Autodesk Inventor part; units mm, degrees
ref_plane "YZ Plane" through (0, 0, 0) normal (1, 0, 0) x (0, 1, 0)
ref_plane "XZ Plane" through (0, 0, 0) normal (0, 1, 0) x (-1, 0, 0)
ref_plane "XY Plane" through (0, 0, 0) normal (0, 0, 1) x (1, 0, 0)
sketch "スケッチ1" plane through (0, 0, 0) normal (0, 0, 1) x (1, 0, 0)
  line L0 (0, 0) -> (239.9998, 0)
  line L1 (239.9998, 0) -> (239.9998, 239.9998)
  line L2 (239.9998, 239.9998) -> (0, 239.9998)
  line L3 (0, 239.9998) -> (0, 0)
  line L4 (0, 239.9998) -> (239.9998, 0)
  line L5 (-178.706, 178.706) -> (151.9787, -151.9787)
  dimension "d16" = 45
  dimension "d17" = 169.7055
extrude "プレート1" add sketch "スケッチ1" along normal blind 1.5 contours L3 L4 L0
sketch "スケッチ2" plane through (0, 0, 1.5) normal (0, 0, 1) x (1, 0, 0)
  line L0 (90, 33.5) -> (110, 33.5)
  line L1 (110, 33.5) -> (110, 86.5)
  line L2 (110, 86.5) -> (90, 86.5)
  line L3 (90, 86.5) -> (90, 33.5)
  line L4 (90, 33.5) -> (110, 86.5) construction
  line L5 (110, 33.5) -> (90, 86.5) construction
  line L6 (239.9998, 0) -> (0, 0)
  line L7 (0, 0) -> (0, 239.9998)
  line L8 (134, 30) -> (66, 30)
  line L9 (66, 30) -> (66, 90)
  line L10 (66, 90) -> (134, 90)
  line L11 (134, 90) -> (134, 30)
  line L12 (134, 30) -> (66, 90) construction
  line L13 (66, 30) -> (134, 90) construction
  point P0 (100, 60)
  dimension "d3" = 20
  dimension "d4" = 53
  dimension "d5" = 60
  dimension "d6" = 100
  dimension "d14" = 60
  dimension "d15" = 68
hole "穴1" at (90, 33.5, 1.5) at (110, 33.5, 1.5) at (90, 86.5, 1.5) at (110, 86.5, 1.5) at (66, 30, 1.5) at (134, 30, 1.5) at (66, 90, 1.5) direction (0, 0, -1) diameter 5.2 depth 1.5 tip angle 118
fillet "フィレット1" radius 2 3 edges at (0, 239.9998, 0.75) (0, 0, 0.75) (239.9998, 0, 0.75)
sketch "スケッチ3" plane through (0, 0, 1.5) normal (0, 0, 1) x (1, 0, 0)
  circle A0 centre (66, 90) radius 2.6
  line L0 (0, 2) -> (0, 235.1714)
  point P0 (0, 0)
  point P1 (90, 117)
  point P2 (80, 117)
  dimension "d19" = 10
  dimension "d20" = 27
  dimension "d21" = 80
hole "穴2" at (90, 117, 1.5) at (80, 117, 1.5) direction (0, 0, -1) diameter 3.242 depth 11.8 tip angle 118
sketch "スケッチ4" plane through (0, 0, 1.5) normal (0, 0, 1) x (1, 0, 0)
  circle A0 centre (90, 117) radius 1.621
  circle A1 centre (80, 117) radius 1.621
  arc A2 (235.1714, 0) -> (236.5856, 3.4142) centre (235.1714, 2) ccw
  line L0 (3.4142, 236.5856) -> (236.5856, 3.4142)
  arc A3 (3.4142, 236.5856) -> (0, 235.1714) centre (2, 235.1714) ccw
  line L1 (0, 2) -> (0, 235.1714)
  arc A4 (0, 2) -> (2, 0) centre (2, 2) ccw
  line L2 (235.1714, 0) -> (2, 0)
  circle A5 centre (134, 30) radius 2.6
  circle A6 centre (110, 86.5) radius 2.6
  circle A7 centre (110, 33.5) radius 2.6
  circle A8 centre (90, 33.5) radius 2.6
  circle A9 centre (90, 86.5) radius 2.6
  circle A10 centre (66, 30) radius 2.6
  circle A11 centre (66, 90) radius 2.6
  line L3 (10, 10) -> (10, 215.8577)
  line L4 (10, 215.8577) -> (215.8577, 10)
  line L5 (215.8577, 10) -> (10, 10)
  point P0 (0, 0)
  point P1 (205, 10)
  point P2 (35, 10)
  point P3 (10, 35)
  point P4 (10, 205)
  point P5 (120, 10)
  point P6 (10, 120)
  dimension "d29" = 10
  dimension "d30" = 25
  dimension "d31" = 25
  dimension "d32" = 170
  dimension "d33" = 170
  dimension "d34" = 85
  dimension "d35" = 85
hole "穴3" at (205, 10, 1.5) at (35, 10, 1.5) at (10, 35, 1.5) at (10, 205, 1.5) at (120, 10, 1.5) at (10, 120, 1.5) direction (0, 0, -1) diameter 4.2 depth 1.5 tip angle 118
sketch "スケッチ6" plane through (0, 0, 1.5) normal (0, 0, 1) x (1, 0, 0)
  circle A0 centre (120, 10) radius 2.1
  circle A1 centre (10, 35) radius 2.1
  circle A2 centre (205, 10) radius 2.1
  circle A3 centre (35, 10) radius 2.1
  circle A4 centre (10, 205) radius 2.1
  circle A5 centre (10, 120) radius 2.1
  circle A6 centre (90, 117) radius 1.621
  circle A7 centre (80, 117) radius 1.621
  arc A8 (235.1714, 0) -> (236.5856, 3.4142) centre (235.1714, 2) ccw
  line L0 (3.4142, 236.5856) -> (236.5856, 3.4142)
  arc A9 (3.4142, 236.5856) -> (0, 235.1714) centre (2, 235.1714) ccw
  line L1 (0, 2) -> (0, 235.1714)
  arc A10 (0, 2) -> (2, 0) centre (2, 2) ccw
  line L2 (235.1714, 0) -> (2, 0)
  circle A11 centre (134, 30) radius 2.6
  circle A12 centre (110, 86.5) radius 2.6
  circle A13 centre (110, 33.5) radius 2.6
  circle A14 centre (90, 33.5) radius 2.6
  circle A15 centre (90, 86.5) radius 2.6
  circle A16 centre (66, 30) radius 2.6
  circle A17 centre (66, 90) radius 2.6
  line L3 (20, 20) -> (20, 191.7155)
  line L4 (20, 191.7155) -> (191.7155, 20)
  line L5 (191.7155, 20) -> (20, 20)
  point P0 (0, 0)
  point P1 (30, 30)
  dimension "d46" = 20
  dimension "d47" = 10
  dimension "d48" = 10
hole "穴4" at (30, 30, 1.5) direction (0, 0, -1) diameter 5.2 depth 1.5 tip angle 118
sketch "スケッチ7" plane through (0, 0, 1.5) normal (0, 0, 1) x (1, 0, 0)
  circle A0 centre (30, 30) radius 2.6
  circle A1 centre (120, 10) radius 2.1
  circle A2 centre (10, 35) radius 2.1
  circle A3 centre (205, 10) radius 2.1
  circle A4 centre (35, 10) radius 2.1
  circle A5 centre (10, 205) radius 2.1
  circle A6 centre (10, 120) radius 2.1
  circle A7 centre (90, 117) radius 1.621
  circle A8 centre (80, 117) radius 1.621
  arc A9 (235.1714, 0) -> (236.5856, 3.4142) centre (235.1714, 2) ccw
  line L0 (3.4142, 236.5856) -> (236.5856, 3.4142)
  arc A10 (3.4142, 236.5856) -> (0, 235.1714) centre (2, 235.1714) ccw
  line L1 (0, 2) -> (0, 235.1714)
  arc A11 (0, 2) -> (2, 0) centre (2, 2) ccw
  line L2 (235.1714, 0) -> (2, 0)
  circle A12 centre (134, 30) radius 2.6
  circle A13 centre (110, 86.5) radius 2.6
  circle A14 centre (110, 33.5) radius 2.6
  circle A15 centre (90, 33.5) radius 2.6
  circle A16 centre (90, 86.5) radius 2.6
  circle A17 centre (66, 30) radius 2.6
  circle A18 centre (66, 90) radius 2.6
  point P0 (0, 0)
extrude "押し出し2" add sketch "スケッチ7" against normal up to surface (1.5 mm away) contours A7 | A8 | A12 | A13 | A14 | A15 | A16 | A17 | A18
equation "\"d12\" = Thickness"
equation "\"d41\" = Thickness"
equation "\"d54\" = Thickness"
equation "\"d2\" = Thickness"
equation "\"BendRadius\" = Thickness"
equation "\"BendReliefWidth\" = Thickness"
equation "\"BendReliefDepth\" = 0.5 * Thickness"
equation "\"CornerReliefSize\" = 4 * Thickness"
equation "\"MinimumRemnant\" = 2 * Thickness"
equation "\"TransitionRadius\" = BendRadius"
equation "\"JacobiRadiusSize\" = BendRadius"
equation "\"GapSize\" = Thickness"
properties part number "Display_CCM_Mount_Top"
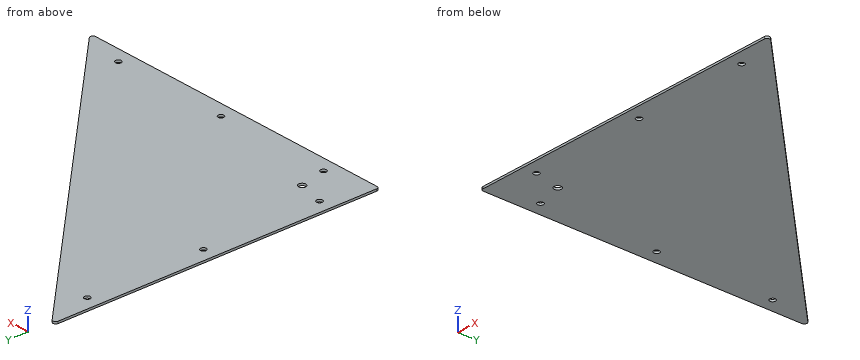
Source: CAD feature listing. Evaluate the final solid. Frame: model axes, mm. Round coordinates to 2 decimals unless told otherwise and drop trailing zeros. Loops run counter-clockwise (first coordinate to the right, second up) from the corner with the lowest first, then second, coordinate; pieces in that order, holes last. Notation, with made-up numbers: (73, 3) - (103, 3) arc R24 ccw to (103, 19) - close; hole circle Ø11 at (21.25, 35). An arc over 180 degrees is marked (long way). Write item = value, one per line. Start each with the question number.
(1) Section query C-C, the plane x = 80. Output: boundary loops of the cut face in (y, z), plus the area to 3 significant figures.
(2) Section query B-B, the plane y = 135.5. Output: boundary loops of the cut face in (x, z), plus the area to 3 significant figures.
(3) Pin query (flat end, axial travel): pin 1 (4 mm diameter, centred on x = 30, y = 30, fed in from +Z). Return the tip coordinate at first contact, or that it passes through.
(4) Ray query, line 1 along Y through (x, z) = (10, 0.3); line 2 along X through (y, z) = (10.5, 0.6); line 3 along X through (y, z) = (32, 1.45). Return the intervals inside material, ascending. Write a range as from..to.
(5) Section query A-A, the plane z = 1.25. Output: boundary loops of the cut face in (x, y), plus the area to 3 significant figures.
Conclusion:
q1.outline = (0, 0) - (160, 0) - (160, 1.5) - (0, 1.5) - close
q1.area = 240 mm2
q2.outline = (0, 0) - (104.5, 0) - (104.5, 1.5) - (0, 1.5) - close
q2.area = 157 mm2
q3.pin_1 = through
q4.line_1 = 0..32.9, 37.1..117.9, 122.1..202.9, 207.1..230
q4.line_2 = 0..32.96, 37.04..117.96, 122.04..202.96, 207.04..229.5
q4.line_3 = 0..28.34, 31.66..208
q5.outline = (0, 2) arc R2 ccw to (2, 0) - (235.17, 0) arc R2 ccw to (236.59, 3.41) - (3.41, 236.59) arc R2 ccw to (0, 235.17) - close; hole circle Ø4.2 at (10, 35); hole circle Ø4.2 at (10, 120); hole circle Ø4.2 at (10, 205); hole circle Ø5.2 at (30, 30); hole circle Ø4.2 at (35, 10); hole circle Ø4.2 at (120, 10); hole circle Ø4.2 at (205, 10)
q5.area = 28,700 mm2
